Model file for the job. Use its own axes, mm. A direction names the side the tool comes from. Round coordinates to 2 decimals unless told otherwise and drop trailing zeros. Order: outer loops, then holes, each group sorted by start corner. A loop starts at its lowest first (then second) coordinate and runs counter-clockwise, first axis right, second up. Notation, with made-up numbers: (-15, -36) - (25, -36) arc R36 ccw to (25, -1) - close; hole circle Ø1 at (75, -1). An arc over 180 degrees is marked (long way). Write item = value, one per line. Start each with the question number.
from build123d import *

# Parameters (mm, degrees)
CROQUIS1_R              = 42.5
SALIENTE_EXTRUIR1_DEPTH = 100
CROQUIS2_R              = 42.5
SALIENTE_EXTRUIR2_DEPTH = 60
CROQUIS3_R              = 42.5
CROQUIS3_R_2            = 36.143595246
CROQUIS3_R_3            = 2.508178933
SALIENTE_EXTRUIR3_DEPTH = 2


with BuildPart() as part:
    # Croquis1 → Saliente-Extruir1 (new body)
    with BuildSketch(Plane(origin=(0, 0, 0), x_dir=(1, 0, 0), z_dir=(0, 1, 0))):
        with Locations(Location((0, 0, 0), (0, 0, 270))):
            Circle(CROQUIS1_R)
    extrude(amount=SALIENTE_EXTRUIR1_DEPTH)

    # Croquis2 → Saliente-Extruir2 (add)
    with BuildSketch(Plane(origin=(0, 0, 0), x_dir=(0, 0, -1), z_dir=(1, 0, 0))):
        with Locations((0, 50)):
            Circle(CROQUIS2_R)
    extrude(amount=SALIENTE_EXTRUIR2_DEPTH)

    # Croquis3 → Saliente-Extruir3 (add)
    with BuildSketch(Plane(origin=(0, 100, 0), x_dir=(1, 0, 0), z_dir=(0, 1, 0))):
        with Locations(Location((0, 0, 0), (0, 0, 270))):
            Circle(CROQUIS3_R)
        with Locations(Location((0, 0, 0), (0, 0, 270))):
            Circle(CROQUIS3_R_2, mode=Mode.SUBTRACT)
        with Locations(Location((0, 39.319059372, 0), (0, 0, 270))):
            Circle(CROQUIS3_R_3, mode=Mode.SUBTRACT)
        with Locations(Location((34.051304269, 19.659529686, 0), (0, 0, 270))):
            Circle(CROQUIS3_R_3, mode=Mode.SUBTRACT)
        with Locations(Location((34.051304269, -19.659529686, 0), (0, 0, 270))):
            Circle(CROQUIS3_R_3, mode=Mode.SUBTRACT)
        with Locations(Location((0, -39.319059372, 0), (0, 0, 270))):
            Circle(CROQUIS3_R_3, mode=Mode.SUBTRACT)
        with Locations(Location((-34.051304269, -19.659529686, 0), (0, 0, 270))):
            Circle(CROQUIS3_R_3, mode=Mode.SUBTRACT)
        with Locations(Location((-34.051304269, 19.659529686, 0), (0, 0, 270))):
            Circle(CROQUIS3_R_3, mode=Mode.SUBTRACT)
    extrude(amount=SALIENTE_EXTRUIR3_DEPTH)


solid = part.part
Item 1: Which spindle directions (+Z, -Z, +X, -X, +Y, -Y) get a long thin tool onto all of the face, cutting with end or side? Do faces 5 (the face through (42.913, 78.724, 31.324)), 6 (the face through (22, 102, -29)), 7 (the face through (31.826, 100.986, -18.502)). Say none if no direction does.
Item 2: Drop flat-ended pins along their axis: pin 1 (3 mm diameter, centred on x = 0, z = -39.32, fed in from +Y); pin 2 (6.5 mm diameter, centred on x = 34.05, z = 19.66, fed in from -Y); pin 3 (2 mm diameter, centred on x = 33.5, y = 44.5, fed in from -Z); pin 4 (3 mm diameter, centred on y = 57.5, z = 28, fed in from -X). Give the stop position or say it passes through.
Item 3: Saw through at A-A, the plane z = 9. Give the cut face in (x, y).
Item 4: Saw through at B-B, the plane x = 5.5. Give the cut face in (y, z).
Item 5: Saw through at D-D, the plane x = -23.5. Give the cut face in (y, z).
Item 6: Saw through at C-C, the plane y = 16. Give the cut face in (x, z), then the cut area to 3 significant figures.
Item 7: Probe L1, parallel to X at y = 100.65, z = 0; L2, parallel to Y at x = -28.5, z = -16; L3, parallel to Z at x = 18.5, y = 48.5. List the from-to ranges inside material, lowest first.
Item 8: Mould opens along X. For faces 1 (the face through (60, 51, 1)), 2 (the face through (-41.49, 50.29, -9.21)), 3 (the face through (-33.298, 100.986, 22.052)), 4 (the face through (34, 100, 20)) say: +X half, -X half, draft (parallel to the pull), parting line (faces both ways), or undercut.
Check sheet entries:
q1.face_5 = +X
q1.face_6 = +Z, -Z, +X, -X, +Y
q1.face_7 = +Y
q2.pin_1 = 100
q2.pin_2 = 0
q2.pin_3 = -42.26
q2.pin_4 = -33.23
q3.outline = (-41.54, 0) - (41.54, 0) - (41.54, 8.46) - (60, 8.46) - (60, 91.54) - (41.54, 91.54) - (41.54, 102) - (35.01, 102) - (35.01, 100) - (-35.01, 100) - (-35.01, 102) - (-41.54, 102) - close
q4.outline = (0, -42.14) - (44.5, -42.14) arc R42.5 ccw to (55.5, -42.14) - (102, -42.14) - (102, -35.72) - (100, -35.72) - (100, 35.72) - (102, 35.72) - (102, 42.14) - (55.5, 42.14) arc R42.5 ccw to (44.5, 42.14) - (0, 42.14) - close
q5.outline = (0, -35.41) - (102, -35.41) - (102, -27.46) - (100, -27.46) - (100, 27.46) - (102, 27.46) - (102, 35.41) - (0, 35.41) - close
q6.outline = (34, -25.5) - (60, -25.5) - (60, 25.5) - (34, 25.5) arc R42.5 ccw (long way) to start
q6.area = 6,710 mm2
q7.L1 = -42.5 to -36.14, 36.14 to 42.5
q7.L2 = 0 to 100
q7.L3 = -42.47 to 42.47
q8.face_1 = +X half
q8.face_2 = parting line
q8.face_3 = undercut
q8.face_4 = undercut
